Check sheet for the drawn part. Datum: minimum x, y, z corner. Units: mm. A direction names the side the tool comes from. Round coordinates to 2 decimals unless told otherwise and drop trailing zeros. Write each loop counter-clockwise with the first axis right and the second up, starting at its lowest first coordinate (ties: lowest second). Pieces come first, ordered by that corner, then holes.
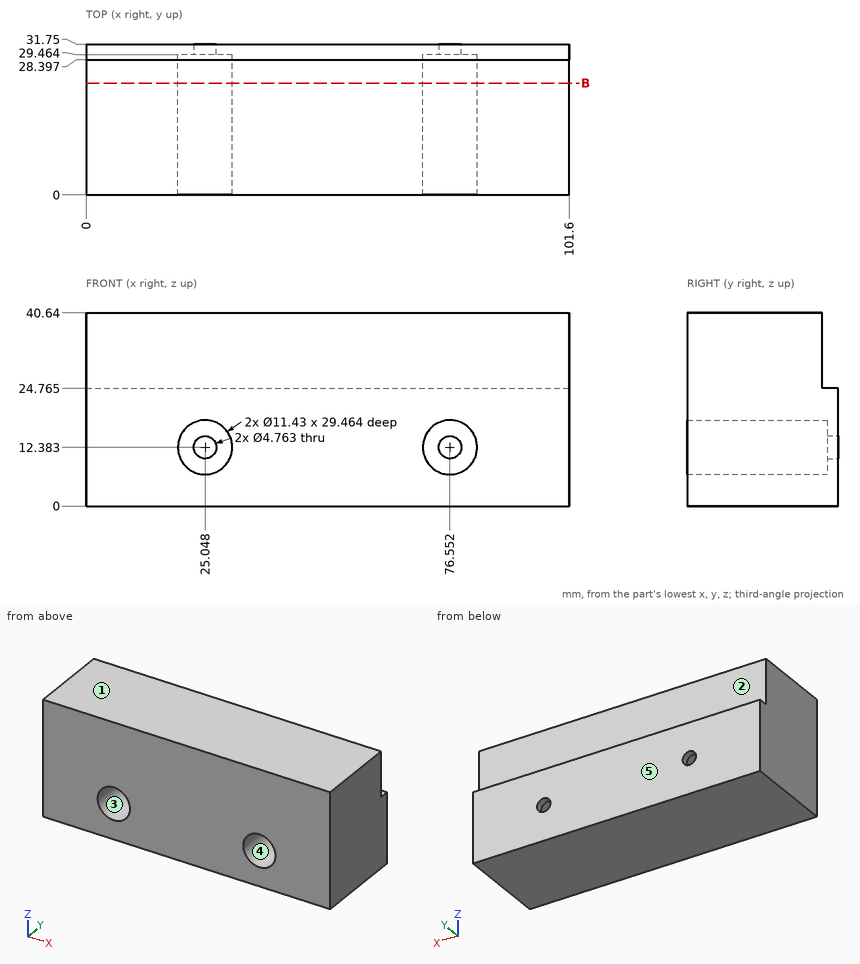
1. Release check for a two-part mould opening along Z. For the marked faces 1, 2 and 3 record: released by +Z, released by -Z, zero draft, split by the parting line, or undercut.
2. Set-up check for the marked faces 4 and 5: record each of +Z, -Z, +X, -X, +Y, -Y from which the full face is reachable in a straight line by a thin tool's end or side.
3. Sectioned sample at B-B, the plane y = 23.5. Enter the section's corners in (x, z) (1 decimal), plus the area to 3 significant figures.
4. Go/stop test with flat-tipped pins: pin 1 (5.5 mm diameter, centred on x = 77.5, z = 14, fed in from -Y); pin 2 (12.5 mm diameter, centred on x = 49.5, z = 34.5, fed in from +Y); pin 3 (1.7 mm diameter, centred on x = 45, y = 29.5, fed in from +Z) (1 decimal); pin 4 (3 mm diameter, centred on x = 76.55, z = 12.38, fed in from +Y). Record where each tip stops, or that it passes through.
5. Scan lines: line 1 along X through (y, z) = (16.5, 11.5) (1 decimal); line 2 along X through (y, z) = (28.5, 14) (1 decimal); line 3 along Z through (x, y) = (20, 16.5) (1 decimal). Record each from-to range of solid material in increasing order.
Computed values:
1. face 1: released by +Z
1. face 2: zero draft
1. face 3: undercut
2. face 4: -Y
2. face 5: +Z, -Z, +X, -X, +Y
3. outline: (0, 0) - (101.6, 0) - (101.6, 40.6) - (0, 40.6) - close; hole circle Ø11.4 at (25, 12.4); hole circle Ø11.4 at (76.6, 12.4)
3. area: 3,920 mm2
4. pin 1: stops at y = 29.46
4. pin 2: stops at y = 28.4
4. pin 3: stops at z = 24.8
4. pin 4: passes through
5. line 1: x = 0 to 19.4, 30.7 to 70.9, 82.2 to 101.6
5. line 2: x = 0 to 19.6, 30.5 to 71.1, 82 to 101.6
5. line 3: z = 0 to 9.7, 15.1 to 40.6
